from build123d import *

# Parameters (mm, degrees)
F0_W     = 45
F0_H     = 45
F0_R     = 17.85
F1_DEPTH = 150
F3_R     = 1.5875
F3_R_2   = 0.813681
F4_DEPTH = 4.3


with BuildPart() as f1:
    # F0 (on Front) → F1 (new body)
    with BuildSketch(Plane.XZ):
        Rectangle(F0_W, F0_H)
        Circle(F0_R, mode=Mode.SUBTRACT)
    extrude(amount=-F1_DEPTH)



with BuildPart() as f4:
    # F3 (on offset) → F4 (new body)
    with BuildSketch(Plane.XZ.offset(25)):
        Circle(F3_R)
        Circle(F3_R_2, mode=Mode.SUBTRACT)
    extrude(amount=-F4_DEPTH)


with BuildPart() as f1_1:
    add(f1.part)

    add(f4.part)  # F6 merges F4
    # F5 (on Right) → F6 (revolve)
    with BuildSketch(Plane.YZ):
        Polygon((-20.7, 0.813681), (0, 17.85), (0, 22.5), (-20.7, 1.5875), align=None)
    revolve(axis=Axis((0, 22.813175, 0), (0, 1, 0)))


solid = f1_1.part
Read the model definition and answer for the solid it produces. Units are mm, in the model's axes. A direction names the side the tool comes from. Give positions to 0.01 mm unless a question says otherwise; leave off trailing zeros. Loops run counter-clockwise (first coordinate to the right, second up) from the corner with the lowest first, then second, coordinate; pieces in that order, holes last. Notation, with made-up numbers: M 87,87 L 102,87 A24 cw 102,116 Z; hole C -4,50.5 d2. An arc over 180 degrees is marked long. Write each question's results on one line, items separated by ' | '.
1. Straight lines are drawn through the part: line 1 (X direction, y = -23, z = 0); line 2 (Z direction, x = 0, y = 106.5). For each, find the intervals that lie inside material, in ascending order. Write a range as [from, to].
Values:
line 1: x = [-1.59, -0.81], [0.81, 1.59] | line 2: z = [-22.5, -17.85], [17.85, 22.5]
2. A tool of negligible diameter and unlimited length cuts with its end or side. For faces 1 (the face through (-18, 0, 17)), 2 (the face through (-18, 0, -17)), 3 (the face through (18, 0, -18)), from which of +Z, -Z, +X, -X, +Y, -Y can it reach the whole face along a straight path? Write none if from no direction.
Values:
face 1: +Z, -X, -Y | face 2: -Z, -X, -Y | face 3: -Z, +X, -Y
3. Given pin 1 (11 mm diameter, centred on x = -9.5, z = 7.5, fed in from -Y); pin 2 (11 mm diameter, centred on x = 12.5, z = 13.5, fed in from -Y); pin 3 (18 mm diameter, centred on x = 16, z = -11.5, fed in from -Y), each flat-ended and moving along its own axis, determine where each tip first touches the part or whether it passes through.
Values:
pin 1: stops at y = -15.73 | pin 2: stops at y = -9.5 | pin 3: stops at y = -11.68
4. Section B-B on y = -13 is taken. Give the vertices of the cut face in (x, z), plus the area to 3 significant figures.
Values:
outline: C 0,0 d18.73; hole C 0,0 d14.3 | area: 115 mm^2
5. Section A-A on y = 105 is taken. Give the vertices of the cut face in (x, z).
Values:
outline: M -22.5,-22.5 L 22.5,-22.5 L 22.5,22.5 L -22.5,22.5 Z; hole C 0,0 d35.7
6. The mould has two halves that part along X. Classify faces 4 (the face through (17, 0, 18)), 5 (the face through (-17.833, 73.95, 0.785)), 6 (the face through (1.48, -17.395, 4.699)): pulls with the +X half, pulls with the -X half, needs draft (parallel to the pull), parting line crosses it, or undercut.
Values:
face 4: needs draft | face 5: undercut | face 6: parting line crosses it
